Here's the drawing with two shaded views (mm, measured from the low corner). I have some questions. A direction names the side the tool comes from. Give positions to 0.01 mm unless a question says otherwise; leave off trailing zeros. Loops run counter-clockwise (first coordinate to the right, second up) from the corner with the lowest first, then second, coordinate; pieces in that order, holes last. Notation, with made-up numbers: (-25, -36.75) - (-5, -36.75) arc R26 ccw to (-5, 2.25) - close; hole circle Ø9 at (5.25, -36.75). An arc over 180 degrees is marked (long way). Use one line per item in the form item = value.
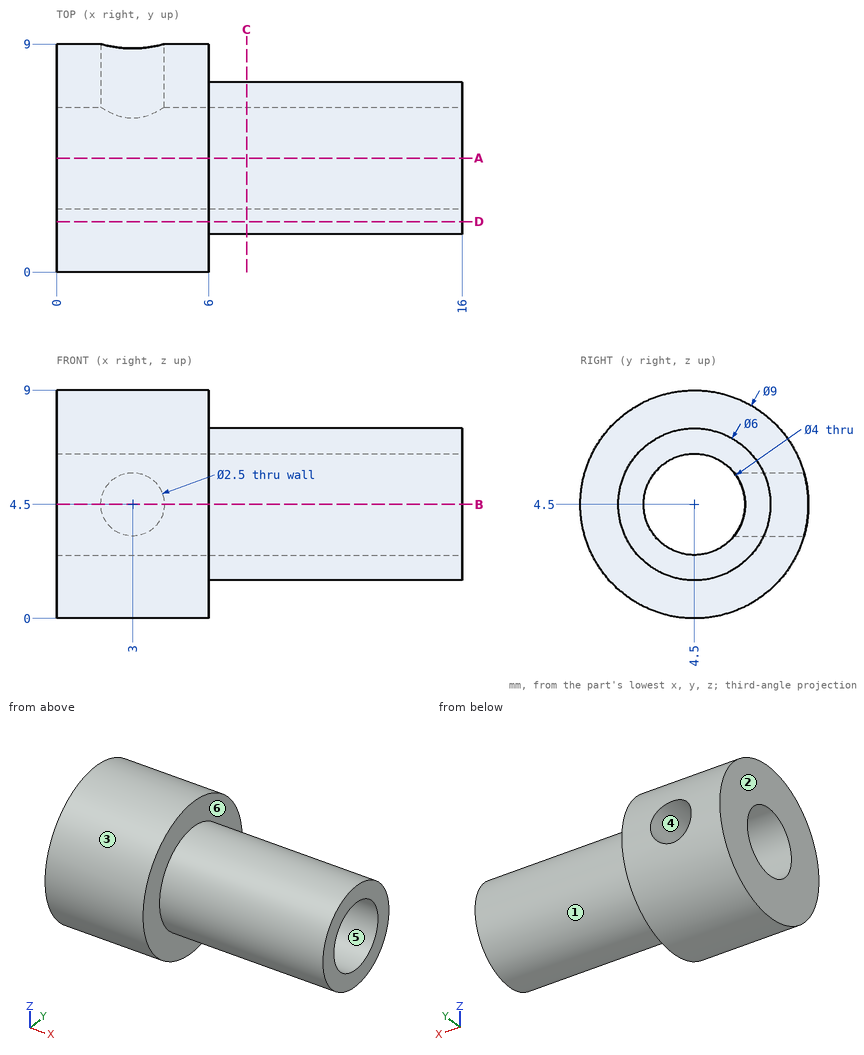
(1) Thinking about a two-plate mould opening in Z: for the marked faces 3, 4, 5 and 6, which applies, pulls with the +Z half, pulls with the -Z half, needs draft (parallel to the pull), parting line crosses it, or undercut?
Geometry says:
face_3 = parting line crosses it
face_4 = undercut
face_5 = undercut
face_6 = needs draft
(2) If we section it at C-C (x = 7.5): List the corners of the cut face in (y, z) for me.
Geometry says:
outline = circle Ø6 at (4.5, 4.5); hole circle Ø4 at (4.5, 4.5)
(3) If we section it at B-B (z = 4.5): List the corners of the cut face in (x, y) for me, plus the area to 4 significant figures.
Geometry says:
outline = (0, 0) - (6, 0) - (6, 1.5) - (16, 1.5) - (16, 2.5) - (0, 2.5) - close; (0, 6.5) - (1.75, 6.5) - (1.75, 9) - (0, 9) - close; (4.25, 6.5) - (16, 6.5) - (16, 7.5) - (6, 7.5) - (6, 9) - (4.25, 9) - close
area = 43.75 mm²
(4) If we section it at D-D (y = 2): List the corners of the cut face in (x, z) for me, plus the area to 3 significant figures.
Geometry says:
outline = (0, 0.76) - (6, 0.76) - (6, 2.84) - (16, 2.84) - (16, 6.16) - (6, 6.16) - (6, 8.24) - (0, 8.24) - close
area = 78.1 mm²
(5) If I drill on probe 1 along Z at (x, y) = (7.75, 4.5); probe 2 along X at (y, z) = (1.5, 4); probe 3 along Y at (x, z) = (5.75, 4.25), over which ranges is the centre line in solid material (lowest first)?
Geometry says:
probe_1 = 1.5 to 2.5, 6.5 to 7.5
probe_2 = 0 to 6
probe_3 = 0.01 to 2.52, 6.48 to 8.99
(6) For P1, Ø2, axis at x = 3, z = 4.5, coming from the +Y side; P2, Ø1, axis at x = 6, z = 3, coming from the +Y side; P3, Ø5, axis at x = 8, y = 2, coming from the +Z side, each with a flat end and sliding along its axis, tell me the tip position at first contact or that it passes through.
Geometry says:
P1 = 2.77
P2 = 8.89
P3 = 8.89
(7) If we section it at A-A (y = 4.5): List the corners of the cut face in (x, z) for me, plus the area to 3 significant figures.
Geometry says:
outline = (0, 0) - (6, 0) - (6, 1.5) - (16, 1.5) - (16, 2.5) - (0, 2.5) - close; (0, 6.5) - (16, 6.5) - (16, 7.5) - (6, 7.5) - (6, 9) - (0, 9) - close
area = 50.0 mm²
(8) For the marked faces 1 and 2, which set-ups out of +Z, -Z, +X, -X, +Y, -Y let a thin tool reach every point of the face, with its end or its side?
Geometry says:
face_1 = +X
face_2 = +Z, -Z, -X, +Y, -Y
